CAD build for the part. Positions are in the model's coordinates, mm. Face numbers are marked on the shaded views. A direction names the side the tool comes from. Round coordinates to 2 decimals unless told otherwise and drop trailing zeros. Order: outer loops, then holes, each group sorted by start corner. A loop starts at its lowest first (then second) coordinate and runs counter-clockwise, first axis right, second up. Notation, with made-up numbers: M -2,47.25 L 39,47.25 A28 ccw 39,68.25 Z; hole C -28,54 d2. An arc over 180 degrees is marked long. Put each result on its own line as item: value.
```python
from build123d import *

# Parameters (mm, degrees)
SKETCH3_W          = 2.667
SKETCH3_H          = 25.4
FILLET1_R          = 3.175
FILLET2_R          = 6.35
CUT_EXTRUDE2_REACH = 27.4
CUT_EXTRUDE3_DEPTH = 3.667


with BuildPart() as part:
    # Sweep1: sweep along a path in Sketch4
    with BuildLine(Plane(origin=(0, 0, 0), x_dir=(1, 0, 0), z_dir=(0, 1, 0))) as sweep1_path:
        Line((0, 0), (0, 31.75))
        Line((0, 31.75), (25.4, 31.75))
    # Sketch3 → Sweep1 (sweep)
    with BuildSketch(Plane.XY):
        with Locations((1.3335, 0)):
            Rectangle(SKETCH3_W, SKETCH3_H)
    sweep(path=sweep1_path.line, transition=Transition.RIGHT)

    # Fillet1
    fillet1_edges = [part.edges().sort_by_distance(p)[0] for p in [
        (2.667, 0, -29.083),
    ]]
    fillet(fillet1_edges, radius=FILLET1_R)

    # Fillet2
    fillet2_edges = [part.edges().sort_by_distance(p)[0] for p in [
        (0, 0, -31.75),
    ]]
    fillet(fillet2_edges, radius=FILLET2_R)

    # Sketch6 → Cut-Extrude2 (cut, up to next)
    with BuildSketch(Plane(origin=(0, 0, 0), x_dir=(0, 0, -1), z_dir=(1, 0, 0)), mode=Mode.PRIVATE) as cut_extrude2_sk1:
        with BuildLine():
            Line((19.558, -3.175), (6.35, -3.175))
            ThreePointArc((6.35, -3.175), (3.175, 0), (6.35, 3.175))
            Line((6.35, 3.175), (19.558, 3.175))
            ThreePointArc((19.558, 3.175), (22.733, 0), (19.558, -3.175))
        make_face()
    cut_extrude2_tool1 = extrude(cut_extrude2_sk1.sketch, amount=CUT_EXTRUDE2_REACH, mode=Mode.PRIVATE) & part.part
    add(cut_extrude2_tool1.solids().sort_by_distance((0, 0, -12.954))[0], mode=Mode.SUBTRACT)

    # Sketch7 → Cut-Extrude3 (cut, through all)
    with BuildSketch(Plane.XY.offset(-29.083)):
        with BuildLine():
            Line((12.192, 3.175), (19.05, 3.175))
            ThreePointArc((19.05, 3.175), (22.225, 0), (19.05, -3.175))
            Line((19.05, -3.175), (12.192, -3.175))
            ThreePointArc((12.192, -3.175), (9.017, 0), (12.192, 3.175))
        make_face()
    extrude(amount=-CUT_EXTRUDE3_DEPTH, mode=Mode.SUBTRACT)


solid = part.part
```
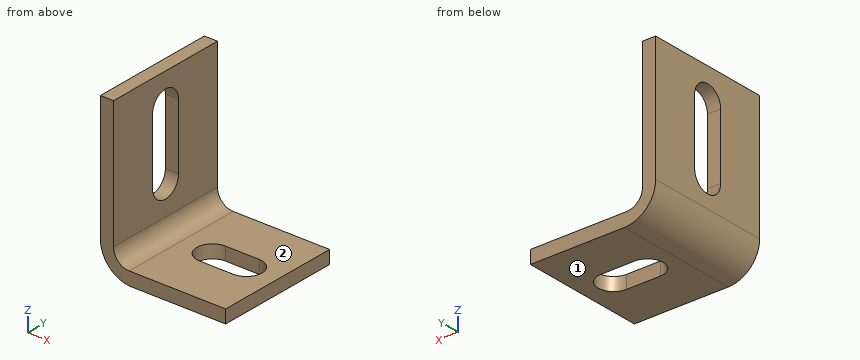
Item 1: Tool access for the marked faces 1 and 2: list every direction of +Z, -Z, +X, -X, +Y, -Y with a clear straight run to the whole face (end or side of a thin tool).
Answers below:
face 1: -Z, +X, -X, +Y, -Y
face 2: +Z, +X, +Y, -Y
Item 2: Probe line 1 along Z through (x, y) = (10.25, -7); line 2 along X through (y, z) = (-9, -4.5); line 3 along Z through (x, y) = (2, -3.5). List the from-to ranges inside material, lowest first. Write a range as [from, to].
Answers below:
line 1: [-31.75, -29.08]
line 2: [0, 2.67]
line 3: [-30.03, 0]
Item 3: Pin check, flat tip, straight feed: P1, Ø1.5, axis at y = 7, z = -18.5, coming from the +X side. Stop position of the tip, or through.
Answers below:
P1: x = 2.67
Item 4: Band-saw the part on C-C on x = 10.5. Give the cut face in (y, z), and give its area (3 significant figures).
Answers below:
outline: M -12.7,-31.75 L -2.69,-31.75 L -2.69,-29.08 L -12.7,-29.08 Z; M 2.69,-31.75 L 12.7,-31.75 L 12.7,-29.08 L 2.69,-29.08 Z
area: 53.4 mm²
Item 5: Band-saw the part on B-B on y = 0. Give the cut face in (x, z) (3 decimals), and give its area (3 significant figures).
Answers below:
outline: M 0,-25.4 A6.35 ccw 6.35,-31.75 L 9.017,-31.75 L 9.017,-29.083 L 5.842,-29.083 A3.175 cw 2.667,-25.908 L 2.667,-22.733 L 0,-22.733 Z; M 0,-3.175 L 2.667,-3.175 L 2.667,0 L 0,0 Z; M 22.225,-31.75 L 25.4,-31.75 L 25.4,-29.083 L 22.225,-29.083 Z
area: 51.4 mm²
Item 6: Band-saw the part on A-A on z = -18.5. Give the cut face in (x, y) (3 decimals), and give its area (3 significant figures).
Answers below:
outline: M 0,-12.7 L 2.667,-12.7 L 2.667,-3.175 L 0,-3.175 Z; M 0,3.175 L 2.667,3.175 L 2.667,12.7 L 0,12.7 Z
area: 50.8 mm²
Item 7: Band-saw the part on D-D on y = 5. Give the cut face in (x, z) (3 decimals).
Answers below:
outline: M 0,-25.4 A6.35 ccw 6.35,-31.75 L 25.4,-31.75 L 25.4,-29.083 L 5.842,-29.083 A3.175 cw 2.667,-25.908 L 2.667,0 L 0,0 Z
